from build123d import *

# Parameters (mm, degrees)
SKETCH_1_W          = 94.8
SKETCH_1_H          = 70
EXTRUDE_1_DEPTH     = 3.2
SKETCH_3_W          = 88.6
SKETCH_3_H          = 63.6
EXTRUDE_2_DEPTH     = 1.5
SKETCH_4_W          = 8
SKETCH_4_H          = 2
EXTRUDE_3_DEPTH     = 6
SKETCH_5_R          = 1.5
CUT_EXTRUDE_1_DEPTH = 100
SKETCH_6_W          = 3
SKETCH_6_H          = 63.6
EXTRUDE_4_DEPTH     = 1.5


with BuildPart() as part:
    # 草图1 → 凸台-拉伸1 (new body)
    with BuildSketch(Plane.XY):
        with Locations((0.1, 0)):
            Rectangle(SKETCH_1_W, SKETCH_1_H)
    extrude(amount=EXTRUDE_1_DEPTH)

    # 草图3 → 凸台-拉伸2 (add)
    with BuildSketch(Plane.XY.offset(3.2)):
        Rectangle(SKETCH_3_W, SKETCH_3_H)
    extrude(amount=EXTRUDE_2_DEPTH)

    # 草图4 → 凸台-拉伸3 (add)
    with BuildSketch(Plane.XY.offset(4.7)):
        with Locations((29.3, 30.8)):
            Rectangle(SKETCH_4_W, SKETCH_4_H)
        with Locations((29.3, -30.8)):
            Rectangle(SKETCH_4_W, SKETCH_4_H)
        with Locations((-29.3, -30.8)):
            Rectangle(SKETCH_4_W, SKETCH_4_H)
        with Locations((-29.3, 30.8)):
            Rectangle(SKETCH_4_W, SKETCH_4_H)
    extrude(amount=EXTRUDE_3_DEPTH)

    # 草图5 → 切除-拉伸1 (cut)
    with BuildSketch(Plane(origin=(0, 31.8, 0), x_dir=(1, 0, 0), z_dir=(0, 1, 0))):
        with Locations(Location((29.3, -7.7, 0), (0, 0, 180))):
            Circle(SKETCH_5_R)
        with Locations(Location((-29.3, -7.7, 0), (0, 0, 180))):
            Circle(SKETCH_5_R)
    extrude(amount=-CUT_EXTRUDE_1_DEPTH, mode=Mode.SUBTRACT)

    # 草图6 → 凸台-拉伸4 (add)
    with BuildSketch(Plane.XY.offset(3.2)):
        with Locations((-45.8, 0)):
            Rectangle(SKETCH_6_W, SKETCH_6_H)
    extrude(amount=EXTRUDE_4_DEPTH)


solid = part.part
Input: part model. Units: mm. Frame: model coordinates. A direction names the side the tool comes from. Give positions to 0.01 mm unless a question says otherwise; leave off trailing zeros. Order: outer loops, then holes, each group sorted by start corner. A loop starts at its lowest first (then second) coordinate and runs counter-clockwise, first axis right, second up. Notation, with made-up numbers: (-13, -29) - (9, -29) arc R26 cw to (9, 8) - close; hole circle Ø4 at (0, 56). An arc over 180 degrees is marked (long way). Answer as a JSON object with one key per item and string values. Group by question number.
Q1. Cut plane B-B, the plane z = 7.7. Count the separate pieces of the cut face and the enclosed holes in it, then the cut area to 3 significant figures.
Q2. Line query: probe 1 along Z at (x, y) = (-29.3, 31.35); probe 2 along Z at (x, y) = (29.5, -20); probe 3 along X at (y, z) = (3, 4.5). Output: solid intervals per line, ascending.
Q3. First-contact query: pin 1 Ø0.8 at (y, z) = (13, 4) entering from +X; pin 2 Ø1.6 at (y, z) = (-31, 9) entering from -X; pin 3 Ø4 at (x, z) = (-29.3, 7.7) entering from -Y; pin 4 Ø2.5 at (x, z) = (29.3, 7.7) entering from -Y. Flat tips, straight axial feed; report the tip coordinate or a pass-through.
Q4. Cut plane D-D, the plane y = -10. Output: boundary loops of the cut face in (x, z).
Q5. Cut plane A-A, the plane x = 29.3. Output: boundary loops of the cut face in (y, z).
Q6. Cut plane C-C, the plane x = -1. Output: boundary loops of the cut face in (y, z), then the cut area to 3 significant figures.
Q7. Set-up query: faces 5 (the face through (33.3, 31, 8)), 6 (the face through (-33.3, 31, 8)), 7 (the face through (-2, -31.8, 4)), 8 (the face through (25.3, -31, 8)). Return all of +Z, -Z, +X, -X, +Y, -Y with unobstructed straight access to the full face (end or side cutting, diameter ignored); none if empty.
Q8. Mould query, pull axis X, two halves, no side actions, for faces 1 (the face through (-30.686, -30.786, 7.125)), 2 (the face through (25.3, 31, 8)), 3 (the face through (-47.3, 0, 2)), 4 (the face through (-1, 35, 2)). Classes: pulls with the +X half, pulls with the -X half, needs draft (parallel to the pull), parting line crosses it, or undercut.
Results:
{
 "1": {"separate pieces": "8", "enclosed holes": "0", "area": "40.0 mm^2"},
 "2": {"probe 1": "0 to 6.2, 9.2 to 10.7", "probe 2": "0 to 4.7", "probe 3": "-47.3 to 44.3"},
 "3": {"pin 1": "x = 44.3", "pin 2": "x = -33.3", "pin 3": "y = -31.8", "pin 4": "through"},
 "4": {"outline": "(-47.3, 0) - (47.5, 0) - (47.5, 3.2) - (44.3, 3.2) - (44.3, 4.7) - (-47.3, 4.7) - close"},
 "5": {"outline": "(-35, 0) - (35, 0) - (35, 3.2) - (31.8, 3.2) - (31.8, 6.2) - (29.8, 6.2) - (29.8, 4.7) - (-29.8, 4.7) - (-29.8, 6.2) - (-31.8, 6.2) - (-31.8, 3.2) - (-35, 3.2) - close; (-31.8, 9.2) - (-29.8, 9.2) - (-29.8, 10.7) - (-31.8, 10.7) - close; (29.8, 9.2) - (31.8, 9.2) - (31.8, 10.7) - (29.8, 10.7) - close"},
 "6": {"outline": "(-35, 0) - (35, 0) - (35, 3.2) - (31.8, 3.2) - (31.8, 4.7) - (-31.8, 4.7) - (-31.8, 3.2) - (-35, 3.2) - close", "area": "319 mm^2"},
 "7": {"face 5": "+Z, +X, +Y, -Y", "face 6": "+Z, -X, +Y, -Y", "face 7": "+Z, +X, -X, -Y", "face 8": "+Z, +Y, -Y"},
 "8": {"face 1": "undercut", "face 2": "undercut", "face 3": "pulls with the -X half", "face 4": "needs draft"}
}
